from build123d import *

# Parameters (mm, degrees)
F0_R     = 37.5
F0_R_2   = 27.5
F1_DEPTH = 20
F2_SIZE  = 3.5
F3_R     = 5


with BuildPart() as f1:
    # F0 (on Top) → F1 (new body)
    with BuildSketch(Plane.XY):
        Circle(F0_R)
        Circle(F0_R_2, mode=Mode.SUBTRACT)
    extrude(amount=F1_DEPTH)

    # F2
    f2_edges = [f1.edges().sort_by_distance(p)[0] for p in [
        (-27.5, 0, 20),
    ]]
    chamfer(f2_edges, length=F2_SIZE)

    # F3
    f3_edges = [f1.edges().sort_by_distance(p)[0] for p in [
        (-37.5, 0, 20),
    ]]
    fillet(f3_edges, radius=F3_R)


solid = f1.part
The listing builds one solid part. Answer for the finished solid, in the listing's coordinates (mm). Coordinates: 2 decimals unless noted, no trailing zeros. Order: outer loops, then holes, each group sorted by start corner. A loop starts at its lowest first (then second) coordinate and runs counter-clockwise, first axis right, second up.
Q1. A cutting plane is placed at A-A, the plane y = 0. Write down the section's boundary in (x, z).
Q2. Given P1, Ø3, axis at x = 4, z = 13.5, coming from the -Y side; P2, Ø8, axis at x = -6.5, z = 2.5, coming from the +Y side; P3, Ø3, axis at y = 14, z = 11.5, coming from the +X side, each flat-ended and moving along its own axis, determine where each tip first touches the part or whether it passes through.
Q3. Consider line 1 (Y direction, x = 0, z = 4.75); line 2 (Y direction, x = -25, z = 9); line 3 (X direction, y = -23, z = 9.25). Determine where each line is inside the solid, lowest interval first.
Q4. A cutting plane is placed at C-C, the plane z = 4.5. Write down the section's boundary in (x, y).
Q5. For a pull along X with two mould halves and no side action, classify faces 1 (the face through (12.79, -24.59, 16.72)), 2 (the face through (-20, 20, 0)), 3 (the face through (-4.88, 37.18, 7.4)), 4 (the face through (-5.961, -26.846, 8.134)) as pulls with the +X half, pulls with the -X half, needs draft (parallel to the pull), parting line crosses it, or undercut.
Q6. A cutting plane is placed at D-D, the plane z = 18.5. Write down the section's boundary in (x, y), and give its area (3 significant figures).
Answers follow:
1. outline: (-37.5, 0) - (-27.5, 0) - (-27.5, 16.5) - (-31, 20) - (-32.5, 20) arc R5 ccw to (-37.5, 15) - close; (27.5, 0) - (37.5, 0) - (37.5, 15) arc R5 ccw to (32.5, 20) - (31, 20) - (27.5, 16.5) - close
2. P1: stops at y = -37.42
2. P2: stops at y = 37.42
2. P3: stops at x = 35.36
3. line 1: y = -37.5 to -27.5, 27.5 to 37.5
3. line 2: y = -27.95 to -11.46, 11.46 to 27.95
3. line 3: x = -29.62 to -15.07, 15.07 to 29.62
4. outline: circle Ø75 at (0, 0); hole circle Ø55 at (0, 0)
5. face 1: undercut
5. face 2: needs draft
5. face 3: parting line crosses it
5. face 4: undercut
6. outline: circle Ø72.14 at (0, 0); hole circle Ø59 at (0, 0)
6. area: 1,350 mm2
